from build123d import *

# Parameters (mm, degrees)
F0_W     = 294.0685
F0_H     = 558.8
F1_DEPTH = 12.7
F3_D     = 4.4
F4_R     = 9.525
F6_DEPTH = 12.701


with BuildPart() as f1:
    # F0 (on Front) → F1 (new body)
    with BuildSketch(Plane.XZ):
        Rectangle(F0_W, F0_H)
    extrude(amount=F1_DEPTH)

    # F3 (through all)
    with Locations(Plane.XZ.offset(12.7)):
        with Locations((-137.50925, 269.875), (-105.75925, 269.875), (105.75925, 269.875), (137.50925, 269.875), (105.75925, -238.125), (137.50925, -238.125), (137.50925, -269.875), (105.75925, -269.875), (-105.75925, -269.875), (-137.50925, -269.875), (-137.50925, -238.125), (-105.75925, -238.125)):
            Hole(F3_D / 2)

    # F4
    f4_edges = [f1.edges().sort_by_distance(p)[0] for p in [
        (147.03425, -6.35, 279.4),
        (147.03425, -6.35, -279.4),
        (-147.03425, -6.35, -279.4),
        (-147.03425, -6.35, 279.4),
    ]]
    fillet(f4_edges, radius=F4_R)

    # F5 (on face) → F6 (cut, through all)
    with BuildSketch(Plane.XZ.offset(12.7)):
        with BuildLine():
            Line((88.9, 241.3), (-88.9, 241.3))
            ThreePointArc((-88.9, 241.3), (-106.8605122421, 233.8605122421), (-114.3, 215.9))
            Line((-114.3, 215.9), (-114.3, -203.2))
            ThreePointArc((-114.3, -203.2), (-106.8605122421, -221.1605122421), (-88.9, -228.6))
            Line((-88.9, -228.6), (88.9, -228.6))
            ThreePointArc((88.9, -228.6), (106.8605122421, -221.1605122421), (114.3, -203.2))
            Line((114.3, -203.2), (114.3, 215.9))
            ThreePointArc((114.3, 215.9), (106.8605122421, 233.8605122421), (88.9, 241.3))
        make_face()
    extrude(amount=-F6_DEPTH, mode=Mode.SUBTRACT)


solid = f1.part
Build history of the part. All positions in model axes, mm. A direction names the side the tool comes from. Give positions to 0.01 mm unless a question says otherwise; leave off trailing zeros. Loops run counter-clockwise (first coordinate to the right, second up) from the corner with the lowest first, then second, coordinate; pieces in that order, holes last. Notation, with made-up numbers: (77.25, 86) - (120.25, 86) arc R24 cw to (120.25, 112) - close; hole circle Ø3 at (7, 76). An arc over 180 degrees is marked (long way). Write item = value, one per line. Start each with the question number.
1) Probe probe 1 along X at (y, z) = (-4.5, 23); probe 2 along Z at (x, y) = (3, -8.75); probe 3 along Z at (x, y) = (106, -1.5). List the from-to ranges inside material, lowest first. Write a range as from..to.
2) Band-saw the part on B-B on x = -47. Give the cut face in (y, z), plus the area to 3 significant figures.
3) Band-saw the part on C-C on y = -5. Count the separate pieces of the cut face and the enclosed holes in it, plus the area to 3 significant figures.
4) Drop a flat-ended pin along its axis: pin 1 Ø5 at (x, z) = (-137.51, -238.12) entering from -Y. Give the stop position or say it passes through.
5) Tool access for faces 5 (the cylindrical face through (-144.318, -6.439, 276.536)), 6 (the cylindrical face through (-106.66, -6.44, 234.06)): list every direction of +Z, -Z, +X, -X, +Y, -Y with a clear straight run to the whole face (end or side of a thin tool).
6) Pull direction X, two halves, no side cores. Call faces 1 (the flat face through (-114.3, -6, 9)), 2 (the flat face through (129, -12.7, 4)), 3 (the flat face through (-147.034, -6, -4)), 4 (the flat face through (114.3, -6, 3)): +X half, -X half, draft (parallel to the pull), parting line (faces both ways), or undercut.
7) Band-saw the part on A-A on z = 83.5. Give the cut face in (x, y).
Final values:
q1.probe_1 = -147.03..-114.3, 114.3..147.03
q1.probe_2 = -279.4..-228.6, 241.3..279.4
q1.probe_3 = -279.4..-272.06, -267.69..-240.31, -235.94..-221.98, 234.68..267.69, 272.06..279.4
q2.outline = (-12.7, -279.4) - (0, -279.4) - (0, -228.6) - (-12.7, -228.6) - close; (-12.7, 241.3) - (0, 241.3) - (0, 279.4) - (-12.7, 279.4) - close
q2.area = 1,130 mm²
q3.separate_pieces = 1
q3.enclosed_holes = 13
q3.area = 57,200 mm²
q4.pin_1 = -12.7
q5.face_5 = +Z, -X, +Y, -Y
q5.face_6 = +Y, -Y
q6.face_1 = undercut
q6.face_2 = draft
q6.face_3 = -X half
q6.face_4 = undercut
q7.outline = (-147.03, -12.7) - (-114.3, -12.7) - (-114.3, 0) - (-147.03, 0) - close; (114.3, -12.7) - (147.03, -12.7) - (147.03, 0) - (114.3, 0) - close
